Autodesk Inventor part; units mm, degrees
ref_plane "YZ Plane" through (0, 0, 0) normal (1, 0, 0) x (0, 1, 0)
ref_plane "XZ Plane" through (0, 0, 0) normal (0, 1, 0) x (-1, 0, 0)
ref_plane "XY Plane" through (0, 0, 0) normal (0, 0, 1) x (1, 0, 0)
sketch "Sketch1" plane through (0, 0, 0) normal (0, 1, 0) x (-1, 0, 0)
  line L0 (0, 0) -> (0, 110)
  line L1 (0, 110) -> (50, 110)
  line L2 (50, 110) -> (50, -110)
  line L3 (50, -110) -> (0, -110)
  line L4 (0, -110) -> (0, 0)
  line L5 (50, 0) -> (0, 0)
  line L6 (50, 110) -> (50, 102.5)
  line L7 (50, 102.5) -> (30, 102.5)
  line L8 (0, 110) -> (-50, 110)
  line L9 (-50, 110) -> (-50, -110)
  line L10 (-50, -110) -> (0, -110)
  circle A0 centre (30, 102.5) radius 3
  line L11 (30, 102.5) -> (-30, 102.5)
  circle A1 centre (-30, 102.5) radius 3
  circle A2 centre (30, -102.5) radius 3
  circle A3 centre (-30, -102.5) radius 3
  line L12 (30, 102.5) -> (30, -102.5)
  line L13 (-30, 102.5) -> (-30, -102.5)
  line L14 (30, 76.2) -> (-30, 50.8) construction
  line L15 (29.0254, 78.5022) -> (-30.9746, 53.1022)
  line L16 (-29.0254, 48.4978) -> (30.9746, 73.8978)
  arc A4 (30.9746, 73.8978) -> (29.0254, 78.5022) centre (30, 76.2) ccw
  arc A5 (-30.9746, 53.1022) -> (-29.0254, 48.4978) centre (-30, 50.8) ccw
  line L17 (30, 50.8) -> (-30, 25.4) construction
  line L18 (29.0254, 53.1022) -> (-30.9746, 27.7022)
  line L19 (-29.0254, 23.0978) -> (30.9746, 48.4978)
  arc A6 (30.9746, 48.4978) -> (29.0254, 53.1022) centre (30, 50.8) ccw
  arc A7 (-30.9746, 27.7022) -> (-29.0254, 23.0978) centre (-30, 25.4) ccw
  line L20 (30, 25.4) -> (-30, 0) construction
  line L21 (29.0254, 27.7022) -> (-30.9746, 2.3022)
  line L22 (-29.0254, -2.3022) -> (30.9746, 23.0978)
  arc A8 (30.9746, 23.0978) -> (29.0254, 27.7022) centre (30, 25.4) ccw
  arc A9 (-30.9746, 2.3022) -> (-29.0254, -2.3022) centre (-30, 0) ccw
  line L23 (30, 0) -> (-30, -25.4) construction
  line L24 (29.0254, 2.3022) -> (-30.9746, -23.0978)
  line L25 (-29.0254, -27.7022) -> (30.9746, -2.3022)
  arc A10 (30.9746, -2.3022) -> (29.0254, 2.3022) centre (30, 0) ccw
  arc A11 (-30.9746, -23.0978) -> (-29.0254, -27.7022) centre (-30, -25.4) ccw
  line L26 (30, -25.4) -> (-30, -50.8) construction
  line L27 (29.0254, -23.0978) -> (-30.9746, -48.4978)
  line L28 (-29.0254, -53.1022) -> (30.9746, -27.7022)
  arc A12 (30.9746, -27.7022) -> (29.0254, -23.0978) centre (30, -25.4) ccw
  arc A13 (-30.9746, -48.4978) -> (-29.0254, -53.1022) centre (-30, -50.8) ccw
  line L29 (30, -50.8) -> (-30, -76.2) construction
  line L30 (29.0254, -48.4978) -> (-30.9746, -73.8978)
  line L31 (-29.0254, -78.5022) -> (30.9746, -53.1022)
  arc A14 (30.9746, -53.1022) -> (29.0254, -48.4978) centre (30, -50.8) ccw
  arc A15 (-30.9746, -73.8978) -> (-29.0254, -78.5022) centre (-30, -76.2) ccw
  point P0 (0, 63.5)
  point P1 (0, 38.1)
  point P2 (0, 12.7)
  point P3 (0, -12.7)
  point P4 (0, -38.1)
  point P5 (0, -63.5)
  dimension "d0" = 110
  dimension "d1" = 50
  dimension "d2" = 220
  dimension "d3" = 7.5
  dimension "d4" = 20
  dimension "d5" = 50
  dimension "d6" = 6
  dimension "d7" = 60
  dimension "d8" = 6
  dimension "d9" = 5
  dimension "d10" = 5
  dimension "d11" = 5
  dimension "d12" = 5
  dimension "d13" = 5
  dimension "d14" = 5
extrude "Extrusion1" add sketch "Sketch1" along normal blind 5 contours L4 L24 L13 A9 L22 L0 | L5 L24 L4 | L0 L22 L12 A10 L24 L5 | L21 L13 A7 L19 L0 | L0 L19 L12 A8 L21 | L22 A8 L12 L19 A6 L16 A4 A0 L7 L2 L5 A10 | L25 L12 A12 L27 L4 | L4 L27 L13 A11 L25 | L24 A11 L13 L27 A13 L30 A15 L31 L4 L10 L9 L8 L0 L11 A1 L15 A5 L18 A7 L21 A9 | L25 A10 L5 L2 L3 L4 L31 A14 L12 L28 A12 | L18 L13 A5 L16 L0 | L0 L16 L12 A6 L18 | L28 L12 A14 L30 L4 | L4 L30 L13 A13 L28 | L7 A0 L11 L0 L1 L2 | L15 L13 A1 L11 L0 | L0 L11 A0 L12 A4 L15
sketch "Sketch2" plane through (0, 5, 0) normal (0, 1, 0) x (1, 0, 0)
  line L0 (-30.9746, -23.0978) -> (29.0254, 2.3022)
  line L1 (29.0254, 2.3022) -> (-30.9746, -23.0978)
  line L2 (30.9746, -2.3022) -> (-29.0254, -27.7022)
  line L3 (30.9746, -2.3022) -> (-29.0254, -27.7022)
  arc A0 (30.9746, -2.3022) -> (29.0254, 2.3022) centre (30, 0) ccw
  arc A1 (30.9746, -2.3022) -> (29.0254, 2.3022) centre (30, 0) ccw
  arc A2 (-30.9746, -23.0978) -> (-29.0254, -27.7022) centre (-30, -25.4) ccw
  arc A3 (-30.9746, -23.0978) -> (-29.0254, -27.7022) centre (-30, -25.4) ccw
  point P0 (0, 0)
extrude "Extrusion2" add sketch "Sketch2" against normal blind 5
sketch "Sketch3" plane through (0, 5, 0) normal (0, 1, 0) x (1, 0, 0)
  line L0 (50, -110) -> (50, 110)
  line L1 (50, 110) -> (50, 0)
  line L2 (50, 0) -> (35, 0)
  circle A0 centre (35, 0) radius 3
  line L3 (-26.3927, -23.0836) -> (18.0573, -4.0336) construction
  line L4 (-25.4079, -25.3815) -> (19.0421, -6.3315)
  line L5 (17.0725, -1.7358) -> (-27.3775, -20.7858)
  arc A1 (-27.3775, -20.7858) -> (-25.4079, -25.3815) centre (-26.3927, -23.0836) ccw
  arc A2 (19.0421, -6.3315) -> (17.0725, -1.7358) centre (18.0573, -4.0336) ccw
  point P0 (0, 0)
  point P1 (-4.1677, -13.5586)
  dimension "d19" = 15
  dimension "d20" = 6
  dimension "d21" = 5
extrude "Extrusion3" cut sketch "Sketch3" against normal blind 5
properties part number "left_side"
Geometry: final body of the model. Coordinates: model frame, mm. A direction names the side the tool comes from. Give positions to 0.01 mm unless a question says otherwise; leave off trailing zeros. Write each loop counter-clockwise with the first axis right and the second up, starting at its lowest first coordinate (ties: lowest second). Pieces come first, ordered by that corner, then holes. Notation, with made-up numbers: (57, 44) -> (73, 44) arc R12 cw to (73, 50) -> close; hole circle Ø8 at (48.5, 28.25). An arc over 180 degrees is marked (long way). Answer as a JSON object with one key per item and string values.
1. Contact query for a flat-ended pin moving along its axis: pin 1 (5.5 mm diameter, centred on x = 35, z = 0, fed in from -Y). Output: stop coordinate, or through.
Ans:
{"pin 1": "passes through"}
2. Cut plane D-D on z = 41. Output: boundary loops of the cut face in (x, y).
Ans:
{"outline": "(-50, 0) -> (-13.26, 0) -> (-13.26, 5) -> (-50, 5) -> close; (-0.44, 0) -> (50, 0) -> (50, 5) -> (-0.44, 5) -> close"}
3. Cut plane B-B on x = 35. Output: boundary loops of the cut face in (y, z), and give its area (3 significant figures).
Ans:
{"outline": "(0, -110) -> (5, -110) -> (5, -3) -> (0, -3) -> close; (0, 3) -> (5, 3) -> (5, 110) -> (0, 110) -> close", "area": "1,070 mm^2"}
4. Ray query, probe 1 along X at (y, z) = (3.55, 102.5); probe 2 along Z at (x, y) = (35, 2.7); probe 3 along X at (y, z) = (4.85, -100). Return the intervals inside material, ascending. Write a range as from..to.
Ans:
{"probe 1": "x = -50..-33, -27..27, 33..50", "probe 2": "z = -110..-3, 3..110", "probe 3": "x = -50..-31.66, -28.34..28.34, 31.66..50"}
5. Mould query, pull axis X, two halves, no side actions, for faces 1 (the flat face through (-1, 2, 110)), 2 (the cylindrical face through (-32.28, 2.465, -49.775)). Classes: pulls with the +X half, pulls with the -X half, needs draft (parallel to the pull), parting line crosses it, or undercut.
Ans:
{"face 1": "needs draft", "face 2": "undercut"}
6. Cut plane C-C on y = 2.45. Count the separate pieces of the cut face and the enclosed holes in it, and give its area (3 significant figures).
Ans:
{"separate pieces": "1", "enclosed holes": "11", "area": "19,900 mm^2"}
7. Access query for faces 3 (the flat face through (0.55, 2.46, -10.22)), 4 (the flat face through (1, 0, 2)). Directions: +Z, -Z, +X, -X, +Y, -Y. A direction counts if a zero-diameter tool reaches every point of the face in a straight line with its end or side. Return the directions, or none.
Ans:
{"face 3": "+Y, -Y", "face 4": "+Z, -Z, +X, -X, -Y"}
8. Cut plane A-A on z = 102.5. Output: boundary loops of the cut face in (x, y), and give its area (3 significant figures).
Ans:
{"outline": "(-50, 0) -> (-33, 0) -> (-33, 5) -> (-50, 5) -> close; (-27, 0) -> (27, 0) -> (27, 5) -> (-27, 5) -> close; (33, 0) -> (50, 0) -> (50, 5) -> (33, 5) -> close", "area": "440 mm^2"}
